Model file for the job. Use its own axes, mm. A direction names the side the tool comes from. Give positions to 0.01 mm unless a question says otherwise; leave off trailing zeros. Order: outer loops, then holes, each group sorted by start corner. A loop starts at its lowest first (then second) coordinate and runs counter-clockwise, first axis right, second up. Notation, with made-up numbers: (82.5, 75.25) - (123.5, 75.25) arc R23 cw to (123.5, 101.25) - close; hole circle Ø8 at (-15, 18). An arc over 180 degrees is marked (long way). Use CSV: the item, a comma, the result in double quotes. Start each with the question number.
(1) Band-saw the part on D-D, the plane y = -0.75. Give the cut face in (x, z) (3 decimals).
(2) Drop flat-ended pins along their axis: pin 1 Ø8 at (x, y) = (10.5, 1.5) entering from -Z; pin 2 Ø8 at (x, y) = (-5, -7) entering from -Z; pin 3 Ø5 at (y, z) = (3, -28) entering from -X. Give the stop position or say it passes through.
(3) Band-saw the part on B-B, the plane z = 0. Give the cut face in (x, y) (1 decimal), then the cut area to 3 significant figures.
(4) Band-saw the part on A-A, the plane x = 0. Give the cut face in (y, z), then the cut area to 3 significant figures.
(5) Tool access for faces 1 (the cylindrical face through (-15.32, 10.12, 11.53)), 2 (the flat face through (0, 0, 23.114)), 3 (the flat face through (5, 10, -25.4)): list every direction of +Z, -Z, +X, -X, +Y, -Y with a clear straight run to the whole face (end or side of a thin tool).
(6) Probe L1, parallel to Y at x = 24.5, z = -4; L2, parallel to X at y = 8, z = 17.5 (3 decimals); L3, parallel to X at y = -10, z = -14.5 (3 decimals). List the from-to ranges inside material, lowest first.
(7) Band-saw the part on C-C, the plane x = 7.5. Give the cut face in (y, z).
(8) Pull direction Z, two halves, no side cores. Call faces 4 (the flat face through (5, -10, -25.4)), 5 (the flat face through (28.575, 0, 0)), 6 (the cylindrical face through (-14.3, 10.12, -11.71)): +Z half, -Z half, draft (parallel to the pull), parting line (faces both ways), or undercut.
from build123d import *

# Parameters (mm, degrees)
SKETCH1_W           = 57.15
SKETCH1_H           = 50.8
BOSS_EXTRUDE1_DEPTH = 11.303
SKETCH2_W           = 52.350000456
SKETCH2_H           = 17.806000456
CUT_EXTRUDE1_DEPTH  = 48.514
SKETCH3_R           = 2.032
SKETCH3_R_2         = 11.1125
CUT_EXTRUDE2_DEPTH  = 2.399999772
SKETCH4_R           = 3.96875
CUT_EXTRUDE3_DEPTH  = 2.399999772
BOSS_EXTRUDE2_REACH = 46.415
SHELL1_START        = -35.538117353
SHELL1_OUTLINE_W    = 14.41756603
SHELL1_OUTLINE_H    = 17.806000456
SHELL1_DEPTH        = 8.538117353
SHELL2_START        = 34.277170944
SHELL2_OUTLINE_W    = 2.993867518
SHELL2_OUTLINE_H    = 17.806000456
SHELL2_DEPTH        = 1.442278976


with BuildPart() as part:
    # Sketch1 → Boss-Extrude1 (new, symmetric)
    with BuildSketch(Plane(origin=(0, 0, 0), x_dir=(1, 0, 0), z_dir=(0, 1, 0))):
        Rectangle(SKETCH1_W, SKETCH1_H)
    extrude(amount=BOSS_EXTRUDE1_DEPTH, both=True)

    # Sketch2 → Cut-Extrude1 (cut)
    with BuildSketch(Plane(origin=(0, 0, -25.4), x_dir=(-1, 0, 0), z_dir=(0, 0, -1))):
        Rectangle(SKETCH2_W, SKETCH2_H)
    extrude(amount=-CUT_EXTRUDE1_DEPTH, mode=Mode.SUBTRACT)

    # Sketch3 → Cut-Extrude2 (cut)
    with BuildSketch(Plane.XZ.offset(11.303)):
        with Locations(Location((-15.494, 15.494, 0), (0, 0, 270))):
            Circle(SKETCH3_R)
        with Locations(Location((15.494, 15.494, 0), (0, 0, 270))):
            Circle(SKETCH3_R)
        with Locations(Location((15.494, -15.494, 0), (0, 0, 270))):
            Circle(SKETCH3_R)
        with Locations(Location((-15.494, -15.494, 0), (0, 0, 270))):
            Circle(SKETCH3_R)
        with Locations(Location((0, 0, 0), (0, 0, 270))):
            Circle(SKETCH3_R_2)
    extrude(amount=-CUT_EXTRUDE2_DEPTH, mode=Mode.SUBTRACT)

    # Sketch4 → Cut-Extrude3 (cut)
    with BuildSketch(Plane(origin=(0, 11.303, 0), x_dir=(1, 0, 0), z_dir=(0, 1, 0))):
        with Locations(Location((-15.494, 15.494, 0), (0, 0, 270))):
            Circle(SKETCH4_R)
        with Locations(Location((15.494, 15.494, 0), (0, 0, 270))):
            Circle(SKETCH4_R)
        with Locations(Location((15.494, -15.494, 0), (0, 0, 270))):
            Circle(SKETCH4_R)
        with Locations(Location((-15.494, -15.494, 0), (0, 0, 270))):
            Circle(SKETCH4_R)
        with Locations(Location((0, 0, 0), (0, 0, 270))):
            Circle(SKETCH4_R)
    extrude(amount=-CUT_EXTRUDE3_DEPTH, mode=Mode.SUBTRACT)

    # Boss-Extrude2: up to this face of the body (flat: up to its plane)
    boss_extrude2_end = Plane(part.part.faces().sort_by_distance((0, -11.303, -24.635358744))[0])
    # Sketch5 → Boss-Extrude2 (add, up to the picked face)
    with BuildSketch(Plane(origin=(0, 11.303, 0), x_dir=(1, 0, 0), z_dir=(0, 1, 0)), mode=Mode.PRIVATE) as boss_extrude2_sk1:
        Polygon((-28.575, 25.4), (-14.097, 25.4), (-14.097, 38.1), align=None)
    boss_extrude2_tool1 = split(extrude(boss_extrude2_sk1.sketch, amount=-BOSS_EXTRUDE2_REACH, mode=Mode.PRIVATE), bisect_by=boss_extrude2_end, keep=Keep.BOTH, mode=Mode.PRIVATE)
    # Sketch5 → Boss-Extrude2 (add, up to the picked face)
    with BuildSketch(Plane(origin=(0, 11.303, 0), x_dir=(1, 0, 0), z_dir=(0, 1, 0)), mode=Mode.PRIVATE) as boss_extrude2_sk2:
        Polygon((28.575, 25.4), (23.749, 25.4), (23.749, 31.75), align=None)
    boss_extrude2_tool2 = split(extrude(boss_extrude2_sk2.sketch, amount=-BOSS_EXTRUDE2_REACH, mode=Mode.PRIVATE), bisect_by=boss_extrude2_end, keep=Keep.BOTH, mode=Mode.PRIVATE)
    add(boss_extrude2_tool1.solids().sort_by(Axis((-18.923, 11.303, -29.633333), (0, -1, 0)))[0])
    add(boss_extrude2_tool2.solids().sort_by(Axis((25.357667, 11.303, -27.516667), (0, -1, 0)))[0])

    # Shell1: read off the stored shape, not the designer's step
    # Shell1 outline → Shell1 (cut)
    with BuildSketch(Plane(origin=(0, 0, 0), x_dir=(0.7517591128712744, 0, -0.6594378183081364), z_dir=(0.6594378183081363, 0, 0.7517591128712744)).offset(SHELL1_START)):
        with Locations((5.21298669, 0)):
            Rectangle(SHELL1_OUTLINE_W, SHELL1_OUTLINE_H)
    extrude(amount=SHELL1_DEPTH, mode=Mode.SUBTRACT)

    # Shell2: read off the stored shape, not the designer's step
    # Shell2 outline → Shell2 (cut)
    with BuildSketch(Plane(origin=(0, 0, 0), x_dir=(0.6050832675335581, 0, 0.7961621941231024), z_dir=(0.7961621941231023, 0, -0.6050832675335583)).offset(SHELL2_START)):
        with Locations((-6.253198947, 0)):
            Rectangle(SHELL2_OUTLINE_W, SHELL2_OUTLINE_H)
    extrude(amount=SHELL2_DEPTH, mode=Mode.SUBTRACT)


solid = part.part
Answer block:
1,outline,"(-28.575, -25.4) - (-14.097, -38.1) - (-14.097, -34.907) - (-24.936, -25.4) - (-26.175, -25.4) - (-26.175, 23.114) - (26.175, 23.114) - (26.175, -25.4) - (25.561, -25.4) - (23.749, -27.784) - (23.749, -31.75) - (28.575, -25.4) - (28.575, 25.4) - (-28.575, 25.4) - close"
2,pin 1,"stops at z = 23.11"
2,pin 2,"stops at z = -25.4"
2,pin 3,"stops at x = -28.46"
3,outline,"(-28.6, -11.3) - (-11.1, -11.3) - (-11.1, -8.9) - (-26.2, -8.9) - (-26.2, 8.9) - (-4, 8.9) - (-4, 11.3) - (-28.6, 11.3) - close; (4, 8.9) - (26.2, 8.9) - (26.2, -8.9) - (11.1, -8.9) - (11.1, -11.3) - (28.6, -11.3) - (28.6, 11.3) - (4, 11.3) - close"
3,area,"287 mm2"
4,outline,"(-11.3, -25.4) - (-8.9, -25.4) - (-8.9, -11.11) - (-11.3, -11.11) - close; (-11.3, 11.11) - (-8.9, 11.11) - (-8.9, 23.11) - (8.9, 23.11) - (8.9, 3.97) - (11.3, 3.97) - (11.3, 25.4) - (-11.3, 25.4) - close; (8.9, -25.4) - (11.3, -25.4) - (11.3, -3.97) - (8.9, -3.97) - close"
4,area,"212 mm2"
5,face 1,"+Y"
5,face 2,"none"
5,face 3,"-Z, +Y, -Y"
6,L1,"y = -11.3 to -8.9, 8.9 to 11.3"
6,L2,"x = -28.575 to -26.175, 26.175 to 28.575"
6,L3,"x = -28.575 to -17.266, -13.722 to 13.722, 17.266 to 28.575"
7,outline,"(-11.3, -25.4) - (-8.9, -25.4) - (-8.9, -8.2) - (-11.3, -8.2) - close; (-11.3, 8.2) - (-8.9, 8.2) - (-8.9, 23.11) - (8.9, 23.11) - (8.9, -25.4) - (11.3, -25.4) - (11.3, 25.4) - (-11.3, 25.4) - close"
8,face 4,"-Z half"
8,face 5,"draft"
8,face 6,"undercut"
